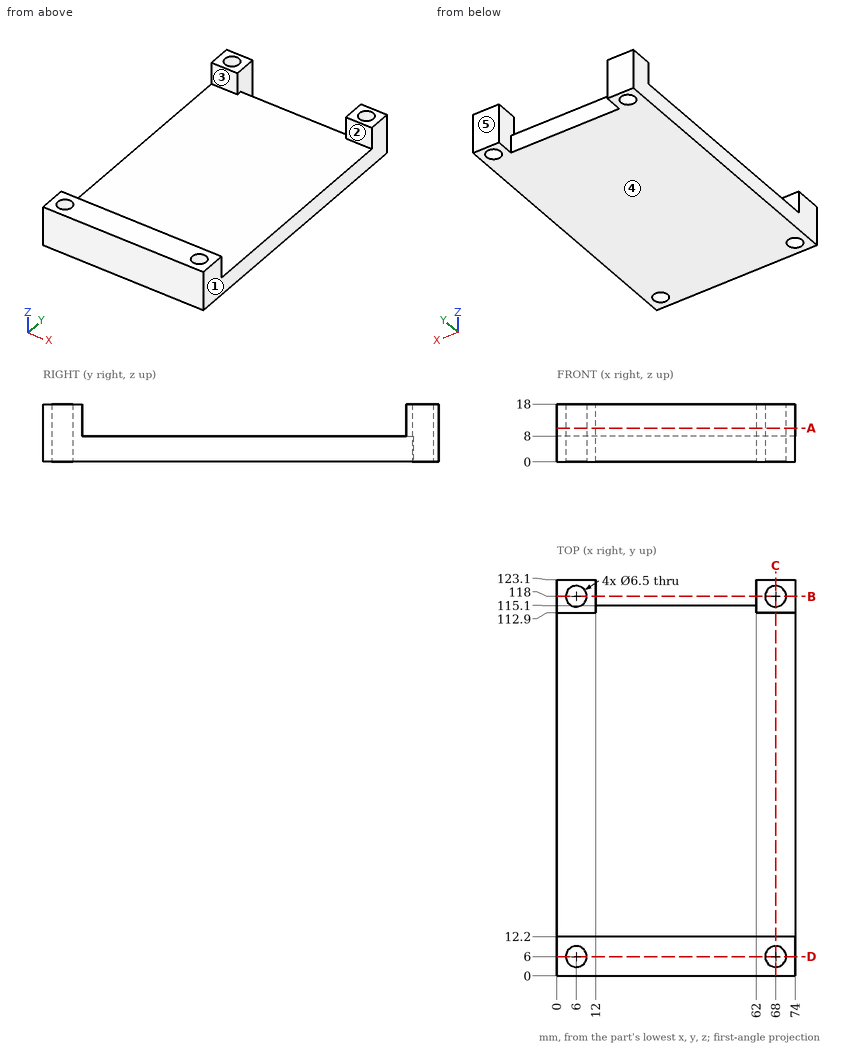
Geometry check sheet. Reference: drawing and pictorial views, mm from the part's lowest x, y, z. A direction names the side the tool comes from. Round coordinates to 2 decimals unless told otherwise and drop trailing zeros. Write each loop counter-clockwise with the first axis right and the second up, starting at its lowest first coordinate (ties: lowest second). Pieces come first, ordered by that corner, then holes.
Item 1: Section check C-C (x = 68). Record the boundary of the cut face in (y, z), plus the area to 3 significant figures.
Determined:
outline: (0, 0) - (2.75, 0) - (2.75, 18) - (0, 18) - close; (9.25, 0) - (114.75, 0) - (114.75, 18) - (112.9, 18) - (112.9, 8) - (12.2, 8) - (12.2, 18) - (9.25, 18) - close; (121.25, 0) - (123.1, 0) - (123.1, 18) - (121.25, 18) - close
area: 975 mm2
Item 2: Access from +Z, -Z, +X, -X, +Y, -Y to the whole of each face (thin tool, end or side, straight path). Record for the marked faces 1 and 2.
Determined:
face 1: +Z, -Z, +X, +Y, -Y
face 2: +Z, +X, -X
Item 3: Section check A-A (z = 10.5). Record the boundary of the cut face in (x, y).
Determined:
outline: (0, 0) - (74, 0) - (74, 12.2) - (0, 12.2) - close; (0, 112.9) - (12, 112.9) - (12, 123.1) - (0, 123.1) - close; (62, 112.9) - (74, 112.9) - (74, 123.1) - (62, 123.1) - close; hole circle Ø6.5 at (6, 6); hole circle Ø6.5 at (6, 118); hole circle Ø6.5 at (68, 6); hole circle Ø6.5 at (68, 118)
Item 4: Section check D-D (y = 6). Record the boundary of the cut face in (x, z).
Determined:
outline: (0, 0) - (2.75, 0) - (2.75, 18) - (0, 18) - close; (9.25, 0) - (64.75, 0) - (64.75, 18) - (9.25, 18) - close; (71.25, 0) - (74, 0) - (74, 18) - (71.25, 18) - close
Item 5: Mould release check, pull along Y, two halves, no side actions. Record for the marked faces 3, 4 and 5: +Y half, -Y half, draft (parallel to the pull), parting line (faces both ways), or undercut.
Determined:
face 3: undercut
face 4: draft
face 5: +Y half
Item 6: Material ranges on line 1 along Y through (x, z) = (6, 8.25); line 2 along Y through (x, z) = (6, 7); line 3 along Y through (x, z) = (42, 16.25), recorded low to high.
Determined:
line 1: y = 0 to 2.75, 9.25 to 12.2, 112.9 to 114.75, 121.25 to 123.1
line 2: y = 0 to 2.75, 9.25 to 114.75, 121.25 to 123.1
line 3: y = 0 to 12.2
Item 7: Section check B-B (y = 118). Record the boundary of the cut face in (x, z).
Determined:
outline: (0, 0) - (2.75, 0) - (2.75, 18) - (0, 18) - close; (9.25, 0) - (12, 0) - (12, 18) - (9.25, 18) - close; (62, 0) - (64.75, 0) - (64.75, 18) - (62, 18) - close; (71.25, 0) - (74, 0) - (74, 18) - (71.25, 18) - close
Item 8: Go/stop test with flat-tipped pins: pin 1 Ø4 at (x, y) = (6, 6) entering from -Z; pin 2 Ø1 at (x, y) = (51.5, 108) entering from +Z; pin 3 Ø6.5 at (x, z) = (34.5, 4.5) entering from +Y. Record where each tip stops, or that it passes through.
Determined:
pin 1: passes through
pin 2: stops at z = 8
pin 3: stops at y = 115.1
